Study the drawing (mm; zero at the part's minimum x, y, z) and answer. Coordinates: 2 decimals unless noted, no trailing zeros. Order: outer loops, then holes, each group sorted by start corner. A loop starts at its lowest first (then second) coordinate and runs counter-clockwise, first axis right, second up. Notation, with made-up numbers: (46.25, 36.25) -> (69.25, 36.25) arc R16 ccw to (69.25, 60.25) -> close; hole circle Ø7 at (61, 68.5). An arc over 180 degrees is marked (long way). Answer in a Markdown table with one row per item. Add a question column.
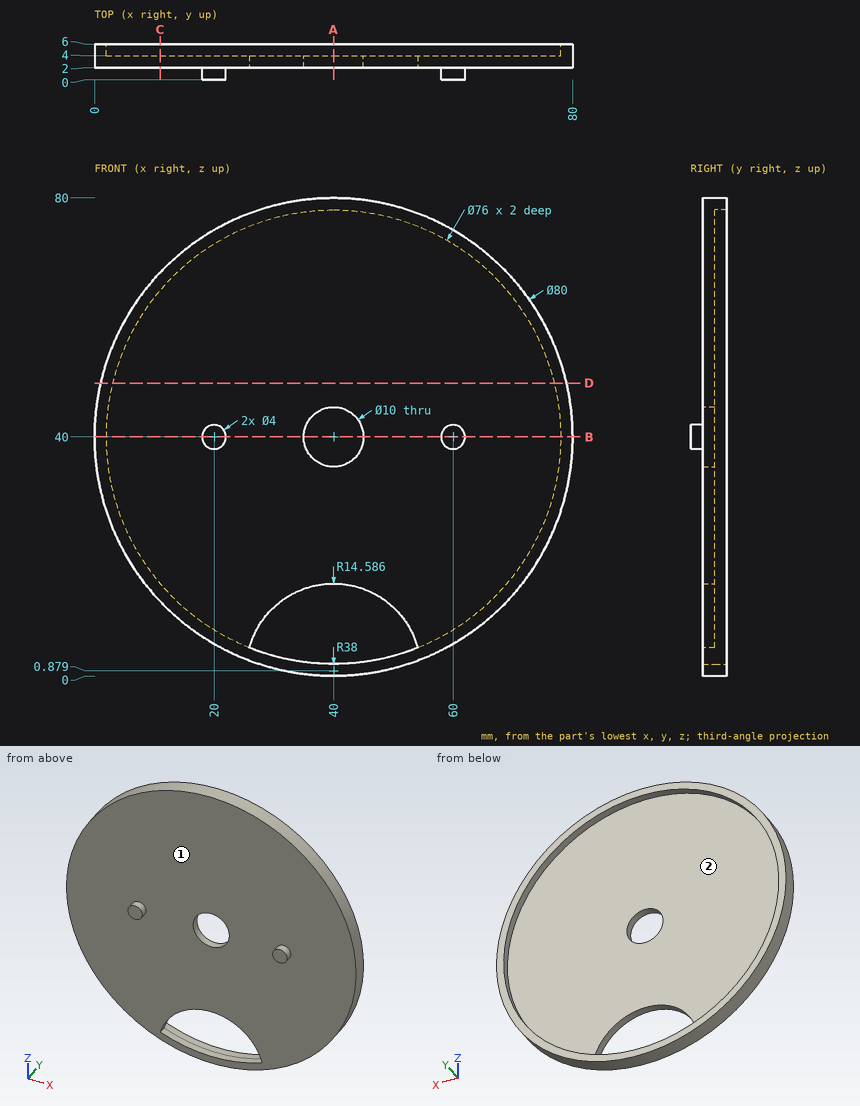
Q1. A cutting plane is placed at A-A (x = 40). Determine the outline of the cut face in (y, z) (1 decimal), then the cut area to 3 significant figures.
Q2. Straight lines are drawn through the part: line 1 (X direction, y = 3.45, z = 40); line 2 (Y direction, x = 23, z = 4.5); line 3 (Y direction, x = 62, z = 38). For each, find the intervals that lie inside material, in ascending order.
Q3. Determine the mould class of the marked faces 1 and 2 for opening direction Z: +Z half, -Z half, draft (parallel to the pull), parting line (faces both ways), or undercut.
Q4. A cutting plane is placed at B-B (z = 40). Determine the outline of the cut face in (x, y).
Q5. Given pin 1 (2 mm diameter, centred on y = 3.5, z = 63, fed in from -X); pin 2 (6 mm diameter, centred on x = 71, z = 43.5, fed in from +Y); pin 3 (2 mm diameter, centred on y = 2, z = 57.5, fed in from -X), each flat-ended and moving along its own axis, determine where each tip first touches the part or whether it passes through.
Q6. A cutting plane is placed at C-C (x = 11). Determine the outline of the cut face in (y, z).
Q7. A cutting plane is placed at D-D (z = 49). Determine the outline of the cut face in (x, y) (1 decimal).
Returned:
| question | item | result |
|---|---|---|
| 1 | outline | (2, 0) -> (6, 0) -> (6, 2) -> (2, 2) -> close; (2, 15.5) -> (4, 15.5) -> (4, 35) -> (2, 35) -> close; (2, 45) -> (4, 45) -> (4, 78) -> (6, 78) -> (6, 80) -> (2, 80) -> close |
| 1 | area | 121 mm² |
| 2 | line 1 | x = 0 to 35, 45 to 80 |
| 2 | line 2 | y = 2 to 6 |
| 2 | line 3 | y = 2 to 4 |
| 3 | face 1 | draft |
| 3 | face 2 | undercut |
| 4 | outline | (0, 2) -> (18, 2) -> (18, 0) -> (22, 0) -> (22, 2) -> (35, 2) -> (35, 4) -> (2, 4) -> (2, 6) -> (0, 6) -> close; (45, 2) -> (58, 2) -> (58, 0) -> (62, 0) -> (62, 2) -> (80, 2) -> (80, 6) -> (78, 6) -> (78, 4) -> (45, 4) -> close |
| 5 | pin 1 | stops at x = 6.59 |
| 5 | pin 2 | stops at y = 4 |
| 5 | pin 3 | stops at x = 3.56 |
| 6 | outline | (2, 12.45) -> (6, 12.45) -> (6, 15.44) -> (4, 15.44) -> (4, 64.56) -> (6, 64.56) -> (6, 67.55) -> (2, 67.55) -> close |
| 7 | outline | (1, 2) -> (79, 2) -> (79, 6) -> (76.9, 6) -> (76.9, 4) -> (3.1, 4) -> (3.1, 6) -> (1, 6) -> close |
